```python
from build123d import *

# Parameters (mm, degrees)
SKETCH2_R          = 8
CUT_EXTRUDE1_DEPTH = 200.283717348
SKETCH3_R          = 4.25
CUT_EXTRUDE2_DEPTH = 18


with BuildPart() as part:
    # Sketch1 → Revolve1 (revolve)
    with BuildSketch(Plane.XY, mode=Mode.PRIVATE) as revolve1_sk:
        Polygon((-22, 0), (-11, 0), (-11, 35.574468085), (-16, 38.334450356), (-16, 52.574533983), (-11, 55.574468085), (-11, 89.856516475), (-22, 97), (-22, 141), (-51, 141), (-51, 136), (-103, 136), (-103, 120), (-54, 120), (-54, 110), (-44, 110), align=None)
    revolve(revolve1_sk.sketch.rotate(Axis((0, 0, 0), (0, 1, 0)), 270), axis=Axis((0, 0, 0), (0, 1, 0)))

    # Sketch2 → Cut-Extrude1 (cut, through all)
    with BuildSketch(Plane(origin=(0, 136, 0), x_dir=(1, 0, 0), z_dir=(0, 1, 0))):
        with Locations(Location((-76, 0, 0), (0, 0, 270))):
            Circle(SKETCH2_R)
        with Locations(Location((-38, 65.817930688, 0), (0, 0, 270))):
            Circle(SKETCH2_R)
        with Locations(Location((38, 65.817930688, 0), (0, 0, 270))):
            Circle(SKETCH2_R)
        with Locations(Location((76, 0, 0), (0, 0, 270))):
            Circle(SKETCH2_R)
        with Locations(Location((38, -65.817930688, 0), (0, 0, 270))):
            Circle(SKETCH2_R)
        with Locations(Location((-38, -65.817930688, 0), (0, 0, 270))):
            Circle(SKETCH2_R)
    extrude(amount=-CUT_EXTRUDE1_DEPTH, mode=Mode.SUBTRACT)

    # Sketch3 → Cut-Extrude2 (cut)
    with BuildSketch(Plane(origin=(0, 141, 0), x_dir=(1, 0, 0), z_dir=(0, 1, 0))):
        with Locations(Location((-38, 0, 0), (0, 0, 270))):
            Circle(SKETCH3_R)
        with Locations(Location((38, 0, 0), (0, 0, 270))):
            Circle(SKETCH3_R)
    extrude(amount=-CUT_EXTRUDE2_DEPTH, mode=Mode.SUBTRACT)


solid = part.part
```
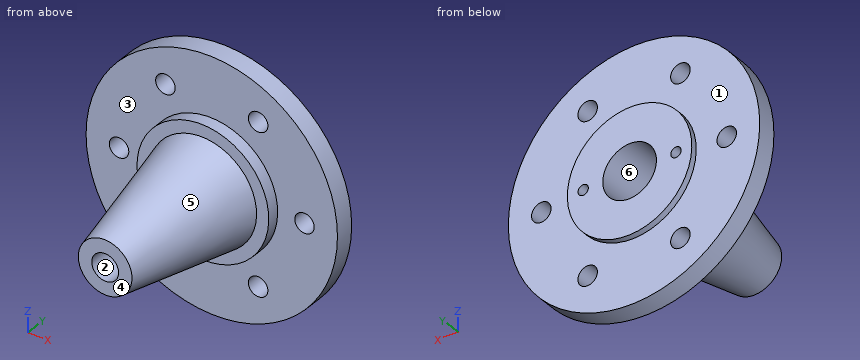
Here's how the part is built. I have some questions about the finished solid (model axes, mm). Face numbers are marked on the shaded views. A direction names the side the tool comes from. Round coordinates to 2 decimals unless told otherwise and drop trailing zeros. Write each loop counter-clockwise with the first axis right and the second up, starting at its lowest first coordinate (ties: lowest second). Pieces come first, ordered by that corner, then holes.
Q1. If we mould it in two halves opening along Z, with no side actions, what happens to the marked faces 4, 5 and 6? For each: +Z half, -Z half, draft (parallel to the pull), parting line (faces both ways), or undercut.
Q2. If we section it at C-C on z = 0: Give the number of separate pieces and of enclosed holes in the cut face, plus the area to 3 significant figures.
Q3. If we section it at A-A on y = 31: Write out the boundary of the cut face in (x, z).
Q4. Will these pins go through, and if not, where does the flat tip stop? P1, Ø6, axis at x = 5, y = 49, coming from the -Z side; P2, Ø21, axis at x = 76, z = 0, coming from the +Y side; P3, Ø10, axis at x = 65.5, z = -71.5, coming from the -Y side.
Q5. Which directions (+Z, -Z, +X, -X, +Y, -Y) give clear straight access to the entire face, cutting with the end or side of a thin tool? Please do the marked faces 1, 2 and 3.
Q6. Please list where these lines run through material, in increasing order: probe 1 along Y at (x, z) = (-62, -62); probe 2 along X at (y, z) = (78.5, 10); probe 3 along Z at (x, y) = (-8.5, 41).
Q7. If we section it at B-B on x = -76: Write out the boundary of the cut face in (y, z).
Answer below:
1. face 4: draft
1. face 5: parting line
1. face 6: undercut
2. separate pieces: 4
2. enclosed holes: 0
2. area: 7,010 mm2
3. outline: circle Ø56.4 at (0, 0); hole circle Ø22 at (0, 0)
4. P1: stops at z = -32.13
4. P2: stops at y = 136
4. P3: stops at y = 120
5. face 1: +Y
5. face 2: +Y, -Y
5. face 3: -Y
6. probe 1: y = 120 to 136
6. probe 2: x = -36.35 to -4.58, 4.58 to 36.35
6. probe 3: z = -28.98 to -13.56, 13.56 to 28.98
7. outline: (120, -69.52) - (136, -69.52) - (136, -8) - (120, -8) - close; (120, 8) - (136, 8) - (136, 69.52) - (120, 69.52) - close
